from build123d import *

# Parameters (mm, degrees)
PAD_DEPTH       = 6
POCKET_DEPTH    = 3
SKETCH002_W     = 18.4
SKETCH002_H     = 20.85
POCKET001_DEPTH = 3
SKETCH003_W     = 8.55
SKETCH003_H     = 1.65
POCKET002_DEPTH = 3


with BuildPart() as part:
    # Sketch → Pad (new body)
    with BuildSketch(Plane.XY):
        with BuildLine():
            ThreePointArc((-75, 28.5), (-103.5, 0), (-75, -28.5))
            Line((-75, -28.5), (75, -28.5))
            ThreePointArc((75, -28.5), (103.5, 0), (75, 28.5))
            Line((-75, 28.5), (75, 28.5))
        make_face()
    extrude(amount=PAD_DEPTH)

    # Sketch001 (on Face6 of Pad) → Pocket (cut)
    with BuildSketch(Plane.XY.offset(6)):
        with BuildLine():
            ThreePointArc((-62.5, 6), (-68.5, 0), (-62.5, -6))
            Line((-62.5, -6), (62.5, -6))
            ThreePointArc((62.5, -6), (68.5, 0), (62.5, 6))
            Line((-62.5, 6), (62.5, 6))
        make_face()
    extrude(amount=-POCKET_DEPTH, mode=Mode.SUBTRACT)

    # Sketch002 (on Face5 of Pocket) → Pocket001 (cut)
    with BuildSketch(Plane.XY.offset(6)):
        with Locations((0, -16.425)):
            Rectangle(SKETCH002_W, SKETCH002_H)
    extrude(amount=-POCKET001_DEPTH, mode=Mode.SUBTRACT)

    # Sketch003 (on Face5 of Pocket001) → Pocket002 (cut)
    with BuildSketch(Plane.XY.offset(6)):
        with Locations((0, -27.675)):
            Rectangle(SKETCH003_W, SKETCH003_H)
    extrude(amount=-POCKET002_DEPTH, mode=Mode.SUBTRACT)


solid = part.part
Build history of the part. All positions in model axes, mm. A direction names the side the tool comes from. Give positions to 0.01 mm unless a question says otherwise; leave off trailing zeros. Loops run counter-clockwise (first coordinate to the right, second up) from the corner with the lowest first, then second, coordinate; pieces in that order, holes last. Notation, with made-up numbers: (39, 9) -> (93, 9) arc R21 cw to (93, 42) -> close; hole circle Ø10 at (-1.5, 36.25). An arc over 180 degrees is marked (long way). Answer in a Markdown table with one row per item.
Item 1: Slice it at A-A on y = 0. Write the cut outline in (x, z), plus the area to 3 significant figures.
Findings below:
| item | result |
|---|---|
| outline | (-103.5, 0) -> (103.5, 0) -> (103.5, 6) -> (68.5, 6) -> (68.5, 3) -> (-68.5, 3) -> (-68.5, 6) -> (-103.5, 6) -> close |
| area | 831 mm² |
Item 2: Mould opens along X. For faces 3 (the cylindrical face through (68.5, -0.1, 4.5)), 4 (the cylindrical face through (103.493, -0.627, 2.958)), 5 (the flat face through (-1, -28.5, 2)), 6 (the cylindrical face through (-103.493, 0.627, 2.958)) say: pulls with the +X half, pulls with the -X half, needs draft (parallel to the pull), parting line crosses it, or undercut.
Findings below:
| item | result |
|---|---|
| face 3 | undercut |
| face 4 | pulls with the +X half |
| face 5 | needs draft |
| face 6 | pulls with the -X half |
Item 3: Slice it at B-B on z = 1.9. Write the cut outline in (x, y), plus the area to 3 significant figures.
Findings below:
| item | result |
|---|---|
| outline | (-75, -28.5) -> (75, -28.5) arc R28.5 ccw to (75, 28.5) -> (-75, 28.5) arc R28.5 ccw to start |
| area | 11,100 mm² |
Item 4: Probe line 1 along Y through (x, z) = (-60, 4.5); line 2 along Y through (x, z) = (9, 5.3); line 3 along X through (y, z) = (1.5, 5.5). List the from-to ranges inside material, lowest first. Write a range as [from, to].
Findings below:
| item | result |
|---|---|
| line 1 | y = [-28.5, -6], [6, 28.5] |
| line 2 | y = [-28.5, -26.85], [6, 28.5] |
| line 3 | x = [-103.46, -68.31], [68.31, 103.46] |
Item 5: Slice it at D-D on y = -25. Write the cut outline in (x, z).
Findings below:
| item | result |
|---|---|
| outline | (-88.68, 0) -> (88.68, 0) -> (88.68, 6) -> (9.2, 6) -> (9.2, 3) -> (-9.2, 3) -> (-9.2, 6) -> (-88.68, 6) -> close |
Item 6: Flat gauge pins, fed straight in: P1, Ø1.5, axis at y = -18, z = 5, coming from the +X side; P2, Ø1.5, axis at y = -18, z = 5, coming from the -X side. Where does each tip first touch, or does it go through?
Findings below:
| item | result |
|---|---|
| P1 | stops at x = 97.69 |
| P2 | stops at x = -97.69 |
Item 7: Tool access for faces 1 (the flat face through (-1, 0, 0)), 2 (the cylindrical face through (-68.5, 0.1, 4.5)): list every direction of +Z, -Z, +X, -X, +Y, -Y with a clear straight run to the whole face (end or side of a thin tool).
Findings below:
| item | result |
|---|---|
| face 1 | -Z, +X, -X, +Y, -Y |
| face 2 | +Z |
Item 8: Slice it at C-C on x = 2. Write the cut outline in (y, z).
Findings below:
| item | result |
|---|---|
| outline | (-28.5, 0) -> (28.5, 0) -> (28.5, 6) -> (6, 6) -> (6, 3) -> (-28.5, 3) -> close |
